from build123d import *

# Parameters (mm, degrees)
SKETCH1_R                       = 17.5
SKETCH1_R_2                     = 5.5
SKETCH1_R_3                     = 1.5
BOSS_EXTRUDE1_DEPTH             = 2
SKETCH1_8_R                     = 5.5
BOSS_EXTRUDE3_DEPTH             = 10
TAP_DRILL_FOR_M2X0_4_TAP1_D     = 2
TAP_DRILL_FOR_M2X0_4_TAP1_DEPTH = 3
TAP_DRILL_FOR_M2X0_4_TAP1_TIP   = 0.600860619


with BuildPart() as part:
    # Sketch1 → Boss-Extrude1 (new body)
    with BuildSketch(Plane.XY):
        Circle(SKETCH1_R)
        Circle(SKETCH1_R_2, mode=Mode.SUBTRACT)
        with Locations((0, 15)):
            Circle(SKETCH1_R_3, mode=Mode.SUBTRACT)
        with Locations((15, 0)):
            Circle(SKETCH1_R_3, mode=Mode.SUBTRACT)
        with Locations((0, -15)):
            Circle(SKETCH1_R_3, mode=Mode.SUBTRACT)
        with Locations((-15, 0)):
            Circle(SKETCH1_R_3, mode=Mode.SUBTRACT)
    extrude(amount=BOSS_EXTRUDE1_DEPTH)

    # Sketch1_8 → Boss-Extrude3 (add)
    with BuildSketch(Plane.XY):
        Circle(SKETCH1_8_R)
    extrude(amount=BOSS_EXTRUDE3_DEPTH)

    # Tap Drill for M2x0.4 Tap1
    with Locations(Plane.XY.offset(10)):
        with Locations((0, 0)):
            Hole(TAP_DRILL_FOR_M2X0_4_TAP1_D / 2, depth=TAP_DRILL_FOR_M2X0_4_TAP1_DEPTH)
            with Locations((0, 0, -(TAP_DRILL_FOR_M2X0_4_TAP1_DEPTH + TAP_DRILL_FOR_M2X0_4_TAP1_TIP / 2))):  # 118° drill point
                Cone(0, TAP_DRILL_FOR_M2X0_4_TAP1_D / 2, TAP_DRILL_FOR_M2X0_4_TAP1_TIP, mode=Mode.SUBTRACT)


solid = part.part
Build history of the part. All positions in model axes, mm. A direction names the side the tool comes from. Coordinates: 2 decimals unless noted, no trailing zeros. Order: outer loops, then holes, each group sorted by start corner. A loop starts at its lowest first (then second) coordinate and runs counter-clockwise, first axis right, second up. Notation, with made-up numbers: (-22, 51.25) - (-14, 51.25) arc R32 ccw to (-14, 78.25) - close; hole circle Ø10 at (27, -19). An arc over 180 degrees is marked (long way). Write each question's results on one line, items separated by ' | '. Start each with the question number.
Item 1: Band-saw the part on D-D on z = 1.5. Write the cut outline in (x, y).
Item 2: Tool access for faces 1 (the face through (-1.19, -5.37, 5.94)), 2 (the face through (-16.5, 0.07, 0.99)): list every direction of +Z, -Z, +X, -X, +Y, -Y with a clear straight run to the whole face (end or side of a thin tool).
Item 3: Band-saw the part on C-C on y = -15. Write the cut outline in (x, z), and give its area (3 significant figures).
Item 4: Band-saw the part on A-A on x = 14. Write the cut outline in (y, z), and give its area (3 significant figures).
Item 5: Wall check: probe 1 along Y at (x, z) = (0, 1.1); probe 2 along Z at (x, y) = (14.5, -2.5); probe 3 along Y at (x, z) = (15, 0.65). Give the ranges that are in metal, low to high. Write a range as [from, to].
Item 6: Flat gauge pins, fed straight in: pin 1 (1.8 mm diameter, centred on x = 0, y = 0, fed in from +Z); pin 2 (4 mm diameter, centred on x = 0, y = -15, fed in from +Z); pin 3 (2.5 mm diameter, centred on x = -15, y = 0, fed in from -Z); pin 4 (1 mm diameter, centred on y = -3, z = 1.5, fed in from +X). Where does each tip first touch, or does it go through?
Item 7: Band-saw the part on B-B on z = 7.75. Write the cut outline in (x, y), and give its area (3 significant figures).
Item 8: Mould opens along X. For faces 3 (the face through (-0.325, -16.464, 0.986)), 4 (the face through (-4, -4, 2)), 5 (the face through (13.5, 0.07, 0.99)), 6 (the face through (-13.887, -10.648, 0.986)) say: released by +X, released by -X, zero draft, split by the parting line, or undercut.
Numbers:
1) outline: circle Ø35 at (0, 0); hole circle Ø3 at (-15, 0); hole circle Ø3 at (0, -15); hole circle Ø3 at (0, 15); hole circle Ø3 at (15, 0)
2) face 1: +Z | face 2: +Z, -Z
3) outline: (-9.01, 0) - (-1.5, 0) - (-1.5, 2) - (-9.01, 2) - close; (1.5, 0) - (9.01, 0) - (9.01, 2) - (1.5, 2) - close | area: 30.1 mm^2
4) outline: (-10.5, 0) - (-1.12, 0) - (-1.12, 2) - (-10.5, 2) - close; (1.12, 0) - (10.5, 0) - (10.5, 2) - (1.12, 2) - close | area: 37.5 mm^2
5) probe 1: [-17.5, -16.5], [-13.5, 13.5], [16.5, 17.5] | probe 2: [0, 2] | probe 3: [-9.01, -1.5], [1.5, 9.01]
6) pin 1: z = 6.94 | pin 2: z = 2 | pin 3: through | pin 4: x = 17.32
7) outline: circle Ø11 at (0, 0); hole circle Ø2 at (0, 0) | area: 91.9 mm^2
8) face 3: undercut | face 4: zero draft | face 5: undercut | face 6: split by the parting line
